```python
from build123d import *

# Parameters (mm, degrees)
SKETCH1_R           = 3.175
SKETCH1_R_2         = 12.7
SKETCH1_R_3         = 1.8161
SKETCH1_R_4         = 7
BOSS_EXTRUDE1_DEPTH = 2.9972
SKETCH2_W           = 2.9972
SKETCH2_H           = 6.35
CUT_EXTRUDE1_DEPTH  = 59.432023179


with BuildPart() as part:
    # Sketch1 → Boss-Extrude1 (new body)
    # profile 1 of 2: a face of its own
    with BuildSketch(Plane.XY):
        with BuildLine():
            Line((-34.05, 9.525), (-12.7, 9.525))
            ThreePointArc((-12.7, 9.525), (0, 22.225), (12.7, 9.525))
            Line((12.7, 9.525), (34.05, 9.525))
            Line((34.05, 9.525), (34.05, 22.225))
            Line((34.05, 22.225), (46.75, 22.225))
            Line((46.75, 22.225), (46.75, 34.925))
            Line((46.75, 34.925), (-46.75, 34.925))
            Line((-46.75, 34.925), (-46.75, 22.225))
            Line((-46.75, 22.225), (-34.05, 22.225))
            Line((-34.05, 22.225), (-34.05, 9.525))
        make_face()
        with Locations(Location((-40.4, 28.575, 0), (0, 0, 180))):
            Circle(SKETCH1_R, mode=Mode.SUBTRACT)
        with Locations(Location((40.4, 28.575, 0), (0, 0, 180))):
            Circle(SKETCH1_R, mode=Mode.SUBTRACT)
    # profile 2 of 2: a face of its own
    with BuildSketch(Plane.XY):
        with Locations((0, 9.525)):
            Circle(SKETCH1_R_2)
        with Locations(Location((0, 0, 0), (0, 0, 180))):
            Circle(SKETCH1_R_3, mode=Mode.SUBTRACT)
        with Locations(Location((0, 9.525, 0), (0, 0, 180))):
            Circle(SKETCH1_R_4, mode=Mode.SUBTRACT)
        with Locations(Location((-8.248891971, 14.2875, 0), (0, 0, 180))):
            Circle(SKETCH1_R_3, mode=Mode.SUBTRACT)
        with Locations(Location((8.248891971, 14.2875, 0), (0, 0, 180))):
            Circle(SKETCH1_R_3, mode=Mode.SUBTRACT)
    extrude(amount=BOSS_EXTRUDE1_DEPTH)

    # Sketch2 → Cut-Extrude1 (cut, through all)
    with BuildSketch(Plane.XY.offset(2.9972)):
        with Locations((-21.8186, 31.75)):
            Rectangle(SKETCH2_W, SKETCH2_H)
        with Locations((21.8186, 31.75)):
            Rectangle(SKETCH2_W, SKETCH2_H)
    extrude(amount=-CUT_EXTRUDE1_DEPTH, mode=Mode.SUBTRACT)


solid = part.part
```
Could you check a few things on this model? Use its own coordinates, in mm. A direction names the side the tool comes from. Round coordinates to 2 decimals unless told otherwise and drop trailing zeros. Loops run counter-clockwise (first coordinate to the right, second up) from the corner with the lowest first, then second, coordinate; pieces in that order, holes last. Notation, with made-up numbers: (6.5, -33.75) - (11.5, -33.75) arc R8 ccw to (11.5, -23.75) - close; hole circle Ø3 at (-24.75, 62). An arc over 180 degrees is marked (long way). Answer as CSV lines item,"result".
1. I want a section at A-A on x = 0. List the corners of the cut face in (y, z) for me (3 decimals).
Filled in:
outline,"(-3.175, 0) - (-1.816, 0) - (-1.816, 2.997) - (-3.175, 2.997) - close; (1.816, 0) - (2.525, 0) - (2.525, 2.997) - (1.816, 2.997) - close; (16.525, 0) - (34.925, 0) - (34.925, 2.997) - (16.525, 2.997) - close"
2. Please list where these lines run through material, in increasing order: line 1 along Y through (x, z) = (0, 1.35) (3 decimals); line 2 along X through (y, z) = (29, 1.1); line 3 along X through (y, z) = (10, 0.8). Write a range as [from, to].
Filled in:
line 1,"y = [-3.175, -1.816], [1.816, 2.525], [16.525, 34.925]"
line 2,"x = [-46.75, -43.55], [-37.25, -23.32], [-20.32, 20.32], [23.32, 37.25], [43.55, 46.75]"
line 3,"x = [-34.05, -6.98], [6.98, 34.05]"
3. I want a section at B-B on y = 6.5. List the corners of the cut face in (x, z) for me.
Filled in:
outline,"(-12.33, 0) - (-6.31, 0) - (-6.31, 3) - (-12.33, 3) - close; (6.31, 0) - (12.33, 0) - (12.33, 3) - (6.31, 3) - close"
4. I want a section at C-C on x = -40.4. List the corners of the cut face in (y, z) for me (3 decimals), then the cut area to 3 significant figures.
Filled in:
outline,"(22.225, 0) - (25.4, 0) - (25.4, 2.997) - (22.225, 2.997) - close; (31.75, 0) - (34.925, 0) - (34.925, 2.997) - (31.75, 2.997) - close"
area,"19.0 mm^2"
5. For pin 1 Ø0.9 at (x, z) = (-24.5, 1.5) entering from -Y (3 decimals); pin 2 Ø1.5 at (x, y) = (16.5, 27.5) entering from -Z, each with a flat end and sliding along its axis, tell me the tip position at first contact or that it passes through.
Filled in:
pin 1,"stops at y = 9.525"
pin 2,"stops at z = 0"
6. We'd pull the mould along Y, two halves only. Please class faces 1 (the face through (46.75, 28, 1)), 2 (the face through (-37.228, 28.435, 1.478)), 3 (the face through (43.572, 28.435, 1.478)), 4 (the face through (35, 34.925, 1)): +Y half, -Y half, draft (parallel to the pull), parting line (faces both ways), or undercut.
Filled in:
face 1,"draft"
face 2,"undercut"
face 3,"undercut"
face 4,"+Y half"
7. I want a section at D-D on y = 30. List the corners of the cut face in (x, z) for me, then the cut area to 3 significant figures.
Filled in:
outline,"(-46.75, 0) - (-43.24, 0) - (-43.24, 3) - (-46.75, 3) - close; (-37.56, 0) - (-23.32, 0) - (-23.32, 3) - (-37.56, 3) - close; (-20.32, 0) - (20.32, 0) - (20.32, 3) - (-20.32, 3) - close; (23.32, 0) - (37.56, 0) - (37.56, 3) - (23.32, 3) - close; (43.24, 0) - (46.75, 0) - (46.75, 3) - (43.24, 3) - close"
area,"228 mm^2"
8. On a 3-axis mill with a long thin cutter (end or side, diameter ignored), from which of +Z, -Z, +X, -X, +Y, -Y can I reach the whole of each face in a straight line? I mean faces 5 (the face through (34.05, 16, 1)), 6 (the face through (23.317, 32, 2)), 7 (the face through (-24, 9.525, 1)). Say none if no direction works.
Filled in:
face 5,"+Z, -Z, +X, -Y"
face 6,"+Z, -Z, +Y"
face 7,"+Z, -Z, -X, -Y"
